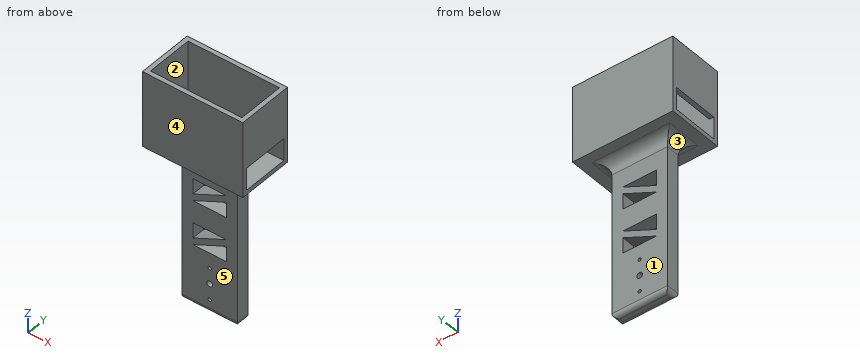
from build123d import *

# Parameters (mm, degrees)
SKETCH1_W           = 25
SKETCH1_H           = 6
BOSS_EXTRUDE1_DEPTH = 70
FILLET1_R           = 2
CUT_EXTRUDE1_DEPTH  = 6
LPATTERN1_COUNT     = 3
LPATTERN1_PITCH     = 20
SKETCH3_W           = 15
SKETCH3_H           = 9.994614872
BOSS_EXTRUDE4_DEPTH = 6
SKETCH4_W           = 45
SKETCH4_H           = 25
BOSS_EXTRUDE5_DEPTH = 2
SKETCH5_W           = 45
SKETCH5_H           = 25
SKETCH5_W_2         = 41
SKETCH5_H_2         = 21
BOSS_EXTRUDE6_DEPTH = 32
FILLET2_R           = 5
SKETCH8_W           = 10
SKETCH8_H           = 21
CUT_EXTRUDE2_DEPTH  = 45
CUT_EXTRUDE3_REACH  = 17.5
SKETCH9_R           = 1.3
SKETCH9_R_2         = 0.75


with BuildPart() as part:
    # Sketch1 → Boss-Extrude1 (new body)
    with BuildSketch(Plane.XY):
        Rectangle(SKETCH1_W, SKETCH1_H)
    extrude(amount=BOSS_EXTRUDE1_DEPTH)

    # Fillet1
    fillet1_edges = [part.edges().sort_by_distance(p)[0] for p in [
        (0, -3, 0),
        (-12.5, 0, 0),
        (0, 3, 0),
        (12.5, 0, 0),
    ]]
    fillet(fillet1_edges, radius=FILLET1_R)

    # Sketch2 → Cut-Extrude1 (cut)
    with BuildSketch(Plane(origin=(0, 3, 0), x_dir=(1, 0, 0), z_dir=(0, 1, 0))):
        Polygon((7.5, -16.994614872), (-7.5, -10), (-7.5, -16.994614872), align=None)
        Polygon((7.5, -13.994614872), (7.5, -7), (-7.5, -7), align=None)
    cut_extrude1 = extrude(amount=-CUT_EXTRUDE1_DEPTH, mode=Mode.SUBTRACT)

    # LPattern1: Cut-Extrude1 ×3
    with Locations(*[(0, 0, i * LPATTERN1_PITCH) for i in range(1, LPATTERN1_COUNT)]):
        add(cut_extrude1, mode=Mode.SUBTRACT)

    # Sketch3 → Boss-Extrude4 (add)
    with BuildSketch(Plane(origin=(0, 3, 0), x_dir=(1, 0, 0), z_dir=(0, 1, 0))):
        with Locations((0, -11.997307436)):
            Rectangle(SKETCH3_W, SKETCH3_H)
    extrude(amount=-BOSS_EXTRUDE4_DEPTH)

    # Sketch4 → Boss-Extrude5 (add)
    with BuildSketch(Plane.XY.offset(70)):
        Rectangle(SKETCH4_W, SKETCH4_H)
    extrude(amount=BOSS_EXTRUDE5_DEPTH)

    # Sketch5 → Boss-Extrude6 (add)
    with BuildSketch(Plane.XY.offset(72)):
        Rectangle(SKETCH5_W, SKETCH5_H)
        Rectangle(SKETCH5_W_2, SKETCH5_H_2, mode=Mode.SUBTRACT)
    extrude(amount=BOSS_EXTRUDE6_DEPTH)

    # Fillet2
    fillet2_edges = [part.edges().sort_by_distance(p)[0] for p in [
        (-12.5, 0, 70),
        (0, -3, 70),
        (12.5, 0, 70),
        (0, 3, 70),
    ]]
    fillet(fillet2_edges, radius=FILLET2_R)

    # Sketch8 → Cut-Extrude2 (cut)
    with BuildSketch(Plane(origin=(22.5, 0, 0), x_dir=(0, 0, -1), z_dir=(1, 0, 0))):
        with Locations((-77, 0)):
            Rectangle(SKETCH8_W, SKETCH8_H)
    extrude(amount=-CUT_EXTRUDE2_DEPTH, mode=Mode.SUBTRACT)

    # Sketch9 → Cut-Extrude3 (cut, up to next)
    with BuildSketch(Plane.XZ.offset(3), mode=Mode.PRIVATE) as cut_extrude3_sk1:
        with Locations((0, 13)):
            Circle(SKETCH9_R)
    cut_extrude3_tool1 = extrude(cut_extrude3_sk1.sketch, amount=-CUT_EXTRUDE3_REACH, mode=Mode.PRIVATE) & part.part
    add(cut_extrude3_tool1.solids().sort_by_distance((0, -3, 13))[0], mode=Mode.SUBTRACT)
    # Sketch9 → Cut-Extrude3 (cut, up to next)
    with BuildSketch(Plane.XZ.offset(3), mode=Mode.PRIVATE) as cut_extrude3_sk2:
        with Locations((0, 20.2)):
            Circle(SKETCH9_R_2)
    cut_extrude3_tool2 = extrude(cut_extrude3_sk2.sketch, amount=-CUT_EXTRUDE3_REACH, mode=Mode.PRIVATE) & part.part
    add(cut_extrude3_tool2.solids().sort_by_distance((0, -3, 20.2))[0], mode=Mode.SUBTRACT)
    # Sketch9 → Cut-Extrude3 (cut, up to next)
    with BuildSketch(Plane.XZ.offset(3), mode=Mode.PRIVATE) as cut_extrude3_sk3:
        with Locations((0, 5.8)):
            Circle(SKETCH9_R_2)
    cut_extrude3_tool3 = extrude(cut_extrude3_sk3.sketch, amount=-CUT_EXTRUDE3_REACH, mode=Mode.PRIVATE) & part.part
    add(cut_extrude3_tool3.solids().sort_by_distance((0, -3, 5.8))[0], mode=Mode.SUBTRACT)


solid = part.part
Work out the finished part from the listing and answer in its coordinate system (mm). Face numbers are marked on the shaded views. A direction names the side the tool comes from. Coordinates: 2 decimals unless noted, no trailing zeros. Write each loop counter-clockwise with the first axis right and the second up, starting at its lowest first coordinate (ties: lowest second). Pieces come first, ordered by that corner, then holes. Notation, with made-up numbers: M 79.5,54.25 L 118.5,54.25 A12 ccw 118.5,66.25 Z; hole C -29.5,39.25 d10. An arc over 180 degrees is marked long. Use one line per item in the form item = value. Start each with the question number.
1. The part is cut by section C-C (x = -9). Give the vertices of the cut face in (y, z), plus the area to 3 significant figures.
2. Straight lines are drawn through the part: probe 1 along Y at (x, z) = (-14, 74); probe 2 along X at (y, z) = (7.25, 95.5); probe 3 along Z at (x, y) = (-19.5, -6.5). For each, find the intervals that lie inside material, in ascending order. Write a range as from..to.
3. The part is cut by section A-A (z = 13). Give the vertices of the cut face in (x, y), plus the area to 3 significant figures.
4. The mould has two halves that part along Y. Classify the marked faces 1, 2 and 3: released by +Y, released by -Y, zero draft, split by the parting line, or undercut.
5. The part is cut by section D-D (z = 32). Give the vertices of the cut face in (x, y), plus the area to 3 significant figures.
6. A tool of negligible diameter and unlimited length cuts with its end or side. For the marked faces 4 and 5, from which of +Z, -Z, +X, -X, +Y, -Y can it reach the whole face along a straight path? Write none if from no direction.
7. The part is cut by section B-B (y = -9). Give the vertices of the cut face in (x, z).
8. Each of these flat-tipped pins is pushed along its axis until it touches: P1, Ø6.5, axis at x = -3, y = 0, coming from the +Z side; P2, Ø10, axis at y = 9, z = 76, coming from the +X side; P3, Ø5, axis at y = -1, z = 30, coming from the -X side; P4, Ø2, axis at x = -22, y = -0.5, coming from the -Z side. Where does it stop, or does it pass through?
Evaluation:
q1.outline = M -12.5,70 L -8,70 A5 cw -3,65 L -3,2 A2 ccw -1,0 L 1,0 A2 ccw 3,2 L 3,65 A5 cw 8,70 L 12.5,70 L 12.5,104 L 10.5,104 L 10.5,72 L -10.5,72 L -10.5,104 L -12.5,104 Z
q1.area = 607 mm^2
q2.probe_1 = -12.5..-10.5, 10.5..12.5
q2.probe_2 = -22.5..-20.5, 20.5..22.5
q2.probe_3 = 70..72
q3.outline = M -12.5,-3 L -1.3,-3 L -1.3,3 L -12.5,3 Z; M 1.3,-3 L 12.5,-3 L 12.5,3 L 1.3,3 Z
q3.area = 134 mm^2
q4.face_1 = released by +Y
q4.face_2 = undercut
q4.face_3 = zero draft
q5.outline = M -12.5,-3 L -7.5,-3 L -7.5,3 L -12.5,3 Z; M -3.21,-3 L 3.22,-3 L 3.22,3 L -3.21,3 Z; M 7.5,-3 L 12.5,-3 L 12.5,3 L 7.5,3 Z
q5.area = 98.6 mm^2
q6.face_4 = +Z, -Z, +X, -X, -Y
q6.face_5 = -Z, +X, -X, -Y
q7.outline = M -22.5,70 L 22.5,70 L 22.5,72 L -22.5,72 Z; M -22.5,82 L -20.5,82 L -20.5,104 L -22.5,104 Z; M 20.5,82 L 22.5,82 L 22.5,104 L 20.5,104 Z
q8.P1 = 72
q8.P2 = 22.5
q8.P3 = -12.5
q8.P4 = 70
